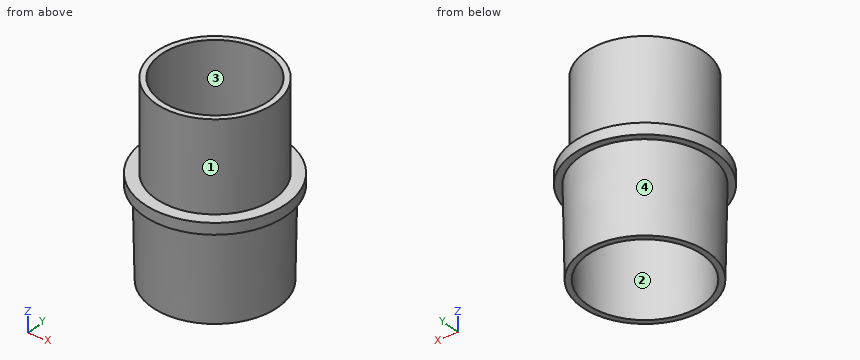
Autodesk Fusion 360 part; units mm, degrees
sketch "Sketch1" plane through (0, 0, 0) normal (0, 0, 1) x (1, 0, 0)
  circle A0 centre (0, 0) radius 28.25
  circle A1 centre (0, 0) radius 25.75
  dimension "d1" = 56.5
  dimension "d7" = 51.5
ref_plane "WorkPlane1" through (0, 0, 40) normal (0, 0, 1) x (1, 0, 0)
sketch "Sketch2" plane through (0, 0, 40) normal (0, 0, 1) x (1, 0, 0)
  circle A0 centre (0, 0) radius 29
  circle A1 centre (0, 0) radius 26.6
  dimension "d6" = 58
  dimension "d8" = 53.2
loft "Loft1" add profiles "Sketch1", "Sketch2" section 1 section 2
loft "Loft2" cut profiles "Sketch2", "Sketch1" section 1 contours A1 section 2 contours A1
sketch "Sketch3" plane through (0, 0, 40) normal (0, 0, 1) x (1, 0, 0)
  circle A0 centre (0, 0) radius 32
  circle A1 centre (0, 0) radius 26.6
  circle A2 centre (0, 0) radius 24.1
  dimension "d9" = 64
  dimension "d10" = 53.2
  dimension "d15" = 48.2
extrude "Extrude1" add sketch "Sketch3" along normal blind 5 contours A0
extrude "Extrude2" add sketch "Sketch3" along normal blind 45 contours A1
Model file for the job. Use its own axes, mm. Face numbers are marked on the shaded views. A direction names the side the tool comes from. Round coordinates to 2 decimals unless told otherwise and drop trailing zeros. Order: outer loops, then holes, each group sorted by start corner. A loop starts at its lowest first (then second) coordinate and runs counter-clockwise, first axis right, second up. Notation, with made-up numbers: M 42,16.25 L 94,16.25 A16 ccw 94,33.25 Z; hole C 16,74.5 d2. An arc over 180 degrees is marked long. Write each question's results on one line, items separated by ' | '. Start each with the question number.
(1) Which spindle directions (+Z, -Z, +X, -X, +Y, -Y) get a long thin tool onto all of the face, cutting with end or side? Do the marked faces 3 and 4. Say none if no direction does.
(2) Saw through at B-B, the plane z = 28. Give the cut face in (x, y) (3 decimals).
(3) Saw through at A-A, the plane z = 57. Give the cut face in (x, y), then the cut area to 3 significant figures.
(4) Two-plate mould, pull along X, no slides. Class the marked faces 1 and 2: pulls with the +X half, pulls with the -X half, needs draft (parallel to the pull), parting line crosses it, or undercut.
(5) Drop flat-ended pins along their axis: pin 1 (2 mm diameter, centred on x = -18, z = 9.5, fed in from -Y); pin 2 (2 mm diameter, centred on x = 19.5, z = 52, fed in from -Y); pin 3 (4 mm diameter, centred on x = -7.5, z = 50, fed in from +Y). Give the stop position or say it passes through.
(6) Probe probe 1 along Y at (x, z) = (0, 75); probe 2 along Y at (x, z) = (11.5, 32.5); probe 3 along Z at (x, y) = (13.5, -26). List the from-to ranges inside material, lowest first. Write a range as from..to.
Established:
1) face 3: +Z, -Z | face 4: -Z
2) outline: C 0,0 d57.55; hole C 0,0 d52.69
3) outline: C 0,0 d53.2; hole C 0,0 d48.2 | area: 398 mm^2
4) face 1: parting line crosses it | face 2: undercut
5) pin 1: stops at y = -22.79 | pin 2: stops at y = -19.11 | pin 3: stops at y = 26.03
6) probe 1: y = -26.6..-24.1, 24.1..26.6 | probe 2: y = -26.47..-23.81, 23.81..26.47 | probe 3: z = 40..45
